```python
from build123d import *
from build123d.topology import SkipClean

# Parameters (mm, degrees)
FILLET_1_R          = 3
SKETCH_2_R          = 2
CUT_EXTRUDE_1_DEPTH = 10


with BuildPart() as part:
    # Sketch 1 → Revolve 1 (revolve)
    with BuildSketch(Plane.XY):
        Polygon((0, -0.4), (0, 16.4), (-6.979971347, 16.4), (-6.979971347, 16.177681197), (-7.205553414, 16.177681197), (-7.205553414, 16.4), (-13.5, 16.4), (-13.5, 0.4), (-24.5, 0.4), (-24.5, -0.4), align=None)
    revolve(axis=Axis((0, 20.6, 0), (0, -1, 0)))

    # Sketch 1_3 → Revolve 2 (revolve)
    with SkipClean():  # the faces are left unmerged after this step: merging them gives an invalid solid
        with BuildSketch(Plane.XY):
            with BuildLine():
                Line((0, 16.4), (6.979971347, 16.4))
                ThreePointArc((6.979971347, 16.4), (4.073082371, 19.4690472), (0, 20.6))
                Line((0, 20.6), (0, 16.4))
            make_face()
            with BuildLine():
                Line((-6.979971347, 16.4), (0, 16.4))
                Line((0, 16.4), (0, 20.6))
                ThreePointArc((0, 20.6), (-4.073082371, 19.4690472), (-6.979971347, 16.4))
            make_face()
        revolve(axis=Axis((0, 20.6, 0), (0, -1, 0)))
    add(part.part.scale(1), mode=Mode.REPLACE)  # the faces are merged on a copy

    # Fillet 1
    fillet_1_edges = [part.edges().sort_by_distance(p)[0] for p in [
        (13.5, 16.4, 0),
    ]]
    fillet(fillet_1_edges, radius=FILLET_1_R)

    # Sketch 2 → Cut-Extrude 1 (cut)
    with BuildSketch(Plane.XZ.offset(0.4)):
        with BuildLine():
            ThreePointArc((21.493704912, 4.90218684), (23.688569985, 2.875293288), (24.5, 0))
            ThreePointArc((24.5, 0), (0, 24.5), (-24.5, 0))
            ThreePointArc((-24.5, 0), (-23.688569985, 2.875293288), (-21.493704912, 4.90218684))
            ThreePointArc((-21.493704912, 4.90218684), (-19.095836123, 6.511883307), (-17.152006375, 8.647866302))
            ThreePointArc((-17.152006375, 8.647866302), (0, 17.502201551), (17.152006375, 8.647866302))
            ThreePointArc((17.152006375, 8.647866302), (19.095836123, 6.511883307), (21.493704912, 4.90218684))
        make_face()
        with BuildLine():
            ThreePointArc((-24.5, 0), (0, -24.5), (24.5, 0))
            ThreePointArc((24.5, 0), (23.688569985, -2.875293288), (21.493704912, -4.90218684))
            ThreePointArc((21.493704912, -4.90218684), (19.095836123, -6.511883307), (17.152006375, -8.647866302))
            ThreePointArc((17.152006375, -8.647866302), (0, -17.502201551), (-17.152006375, -8.647866302))
            ThreePointArc((-17.152006375, -8.647866302), (-19.095836123, -6.511883307), (-21.493704912, -4.90218684))
            ThreePointArc((-21.493704912, -4.90218684), (-23.688569985, -2.875293288), (-24.5, 0))
        make_face()
        with Locations((-19, 0)):
            Circle(SKETCH_2_R)
        with Locations((19, 0)):
            Circle(SKETCH_2_R)
    extrude(amount=-CUT_EXTRUDE_1_DEPTH, mode=Mode.SUBTRACT)


solid = part.part
```
Could you check a few things on this model? Use its own coordinates, in mm. A direction names the side the tool comes from. Give positions to 0.01 mm unless a question says otherwise; leave off trailing zeros. Loops run counter-clockwise (first coordinate to the right, second up) from the corner with the lowest first, then second, coordinate; pieces in that order, holes last. Notation, with made-up numbers: (5, 85) - (52, 85) arc R17 ccw to (52, 100) - close; hole circle Ø11 at (70, -5). An arc over 180 degrees is marked (long way). Use one line per item in the form item = value.
1. I need wall thicknesses on probe 1 along Z at (x, y) = (-19, -0.15); probe 2 along X at (y, z) = (11.5, -8.5); probe 3 along Y at (x, z) = (-1.5, -9). Which ranges of each line are inside material? Lowest first, please.
Response values:
probe_1 = -6.6 to -2, 2 to 6.6
probe_2 = -10.49 to 10.49
probe_3 = -0.4 to 16.4
2. On a 3-axis mill with a long thin cutter (end or side, diameter ignored), from which of +Z, -Z, +X, -X, +Y, -Y can I reach the whole of each face in a straight line? I mean faces 4 (the face through (-0.3, 0, 17.5)), 5 (the face through (7, 0.4, -12)). Say none if no direction works.
Response values:
face_4 = +Z, +Y, -Y
face_5 = +Y
3. I'm going to push flat-ended pins straight in: pin 1 Ø2 at (x, z) = (9, 10) entering from +Y; pin 2 Ø6.5 at (x, z) = (19, 0) entering from -Y; pin 3 Ø3 at (x, y) = (-8, 8.5) entering from -Z; pin 4 Ø5 at (x, y) = (-17, 13.5) entering from +Z. Where does each tip first touch, or does it pass through?
Response values:
pin_1 = 15.68
pin_2 = -0.4
pin_3 = -11.83
pin_4 = through
4. I want a section at B-B (x = 0). Please give me the cut outline in (y, z), and give its area (3 significant figures).
Response values:
outline = (-0.4, -17.5) - (0.4, -17.5) - (0.4, -13.5) - (13.4, -13.5) arc R3 ccw to (16.4, -10.5) - (16.4, -7.21) - (16.18, -7.21) - (16.18, -6.98) - (16.4, -6.98) arc R7.9 ccw to (16.4, 6.98) - (16.18, 6.98) - (16.18, 7.21) - (16.4, 7.21) - (16.4, 10.5) arc R3 ccw to (13.4, 13.5) - (0.4, 13.5) - (0.4, 17.5) - (-0.4, 17.5) - close
area = 498 mm²
5. I want a section at A-A (x = 19). Please give me the cut outline in (y, z).
Response values:
outline = (-0.4, -6.6) - (0.4, -6.6) - (0.4, -2) - (-0.4, -2) - close; (-0.4, 2) - (0.4, 2) - (0.4, 6.6) - (-0.4, 6.6) - close
6. I want a section at C-C (y = 17.25). Please give me the cut outline in (x, z), and give its area (3 significant figures).
Response values:
outline = circle Ø12.92 at (0, 0)
area = 131 mm²
7. Thinking about a two-plate mould opening in Z: for faces 1 (the face through (-19.065, -0.006, -6.538)), 2 (the face through (0, -0.4, 0)), 3 (the face through (-20.6, 0, -1.2)), which applies, released by +Z, released by -Z, zero draft, split by the parting line, or undercut?
Response values:
face_1 = released by -Z
face_2 = zero draft
face_3 = undercut
